CAD build for the part. Positions are in the model's coordinates, mm. A direction names the side the tool comes from. Round coordinates to 2 decimals unless told otherwise and drop trailing zeros. Loops run counter-clockwise (first coordinate to the right, second up) from the corner with the lowest first, then second, coordinate; pieces in that order, holes last.
Autodesk Inventor part; units mm, degrees
ref_plane "YZ Plane" through (0, 0, 0) normal (1, 0, 0) x (0, 1, 0)
ref_plane "XZ Plane" through (0, 0, 0) normal (0, 1, 0) x (-1, 0, 0)
ref_plane "XY Plane" through (0, 0, 0) normal (0, 0, 1) x (1, 0, 0)
sketch "Sketch1" plane through (0, 0, 0) normal (0, 0, 1) x (1, 0, 0)
  line L0 (0, 0) -> (0, 9.525)
  line L1 (0, 9.525) -> (3.7084, 9.525)
  line L2 (3.7084, 9.525) -> (3.7084, 3.9751)
  line L3 (3.7084, 3.9751) -> (23.5458, 3.9751)
  line L4 (23.5458, 3.9751) -> (23.5458, 2.413)
  line L5 (23.5458, 2.413) -> (33.1978, 2.413)
  line L6 (33.1978, 2.413) -> (33.1978, 0)
  line L7 (33.1978, 0) -> (0, 0)
  dimension "d0" = 9.525
  dimension "d1" = 3.9751
  dimension "d2" = 3.7084
  dimension "d3" = 9.652
  dimension "d4" = 33.1978
  dimension "d5" = 2.413
revolve "Revolution1" add sketch "Sketch1" angle 360 about axis through (33.1978, 0, 0) along (-1, 0, 0)
thread "Thread1"
properties part number "Pancake Shifter Shaft"
Item 1: Cut at C-C, the plane x = 21. Give the cut face in (y, z).
Answers follow:
outline: circle Ø7.95 at (0, 0)
Item 2: Probe line 1 (X direction, y = 7, z = -5.5); line 2 (X direction, y = -0.5, z = 3.75); line 3 (Z direction, x = 18, y = -0.25). List the from-to ranges inside material, lowest first.
Answers follow:
line 1: x = 0 to 3.71
line 2: x = 0 to 23.55
line 3: z = -3.97 to 3.97
Item 3: Flat gauge pins, fed straight in: P1, Ø8, axis at x = 21, z = -1, coming from the -Y side; P2, Ø4, axis at x = 27, y = 2, coming from the +Z side; P3, Ø8, axis at x = 20, y = -5, coming from the -Z side. Where does each tip first touch, or does it go through?
Answers follow:
P1: stops at y = -3.98
P2: stops at z = 2.41
P3: stops at z = -3.85
Item 4: Cut at A-A, the plane y = 0. Give the cut face in (x, z) (3 decimals).
Answers follow:
outline: (0, -9.525) - (3.708, -9.525) - (3.708, -3.975) - (23.546, -3.975) - (23.546, -2.413) - (33.198, -2.413) - (33.198, 2.413) - (23.546, 2.413) - (23.546, 3.975) - (3.708, 3.975) - (3.708, 9.525) - (0, 9.525) - close
Item 5: Cut at D-D, the plane x = 31. Give the cut face in (y, z).
Answers follow:
outline: circle Ø4.83 at (0, 0)
Item 6: 3-axis set-ups, long thin cutter, end or side, ignore diameter. For faces 1 (the cylindrical face through (28.439, -1.915, -1.468)), 2 (the flat face through (0, 0, 0)): which of +Z, -Z, +X, -X, +Y, -Y reach the whole face in a straight line?
Answers follow:
face 1: +X
face 2: +Z, -Z, -X, +Y, -Y
